```python
from build123d import *

# Parameters (mm, degrees)
BOX001_W               = 7.07
BOX001_H               = 20
BOX001_DEPTH           = 7.07
BOX001_PLACEMENT_ANGLE = 45
BOX_W                  = 10
BOX_H                  = 20
BOX_DEPTH              = 10


with BuildPart() as cubo001:
    # Box001 → Box001 (new body)
    with BuildSketch(Plane.XY):
        with Locations((3.535, 10)):
            Rectangle(BOX001_W, BOX001_H)
    extrude(amount=BOX001_DEPTH)


with BuildPart() as cubo001_1:
    # Box001 placement: moved
    add(cubo001.part.moved(Location((-5, -10, 10))).rotate(Axis((-5, -10, 10), (0, 1, 0)), BOX001_PLACEMENT_ANGLE))


with BuildPart() as fusion:
    # Box → Box (new body)
    with BuildSketch(Plane(origin=(-5, -10, 0), x_dir=(1, 0, 0), z_dir=(0, 0, 1))):
        with Locations((5, 10)):
            Rectangle(BOX_W, BOX_H)
    extrude(amount=BOX_DEPTH)

    # Fusion: union Cubo001
    add(cubo001_1.part)


solid = fusion.part
```
For this review, take the finished solid that the model builds, in its own axes (mm). Coordinates: 2 decimals unless noted, no trailing zeros. Write each loop counter-clockwise with the first axis right and the second up, starting at its lowest first coordinate (ties: lowest second). Pieces come first, ordered by that corner, then holes. Notation, with made-up numbers: (57.5, 31) - (110.5, 31) arc R27 cw to (110.5, 67) - close; hole circle Ø1 at (-25.75, -36). An arc over 180 degrees is marked (long way). Answer in a Markdown table with one row per item. Add a question column.
Q1. We need section C-C, the plane z = 14. State the section outline as (x, y) points, and give its area (3 significant figures).
Q2. For probe 1 along X at (y, z) = (-8, 11); probe 2 along Z at (x, y) = (-4, -3.5); probe 3 along Z at (x, y) = (-2, 7), list the stretches that pass through material, from the lowest coordinate up.
Q3. We need section A-A, the plane x = -2.25. State the section outline as (y, z) points.
Q4. For P1, Ø3, axis at x = 2.5, y = 3, coming from the +Z side, flat-tipped, find the tip position at first contact; note if it passes through.
Answer list:
| question | item | result |
|---|---|---|
| 1 | outline | (-1, -10) - (1, -10) - (1, 10) - (-1, 10) - close |
| 1 | area | 40.0 mm2 |
| 2 | probe 1 | x = -4 to 4 |
| 2 | probe 2 | z = 0 to 11 |
| 2 | probe 3 | z = 0 to 13 |
| 3 | outline | (-10, 0) - (10, 0) - (10, 12.75) - (-10, 12.75) - close |
| 4 | P1 | stops at z = 14 |
